Verification items for this drawing (mm, ordinates from the low corner). A direction names the side the tool comes from. Round coordinates to 2 decimals unless told otherwise and drop trailing zeros. Write each loop counter-clockwise with the first axis right and the second up, starting at its lowest first coordinate (ties: lowest second). Pieces come first, ordered by that corner, then holes. Notation, with made-up numbers: (-38.75, 71) -> (12.25, 71) arc R13 cw to (12.25, 94) -> close; hole circle Ø7 at (45.5, -5). An arc over 180 degrees is marked (long way). Put each result on its own line as item: value. Start each with the question number.
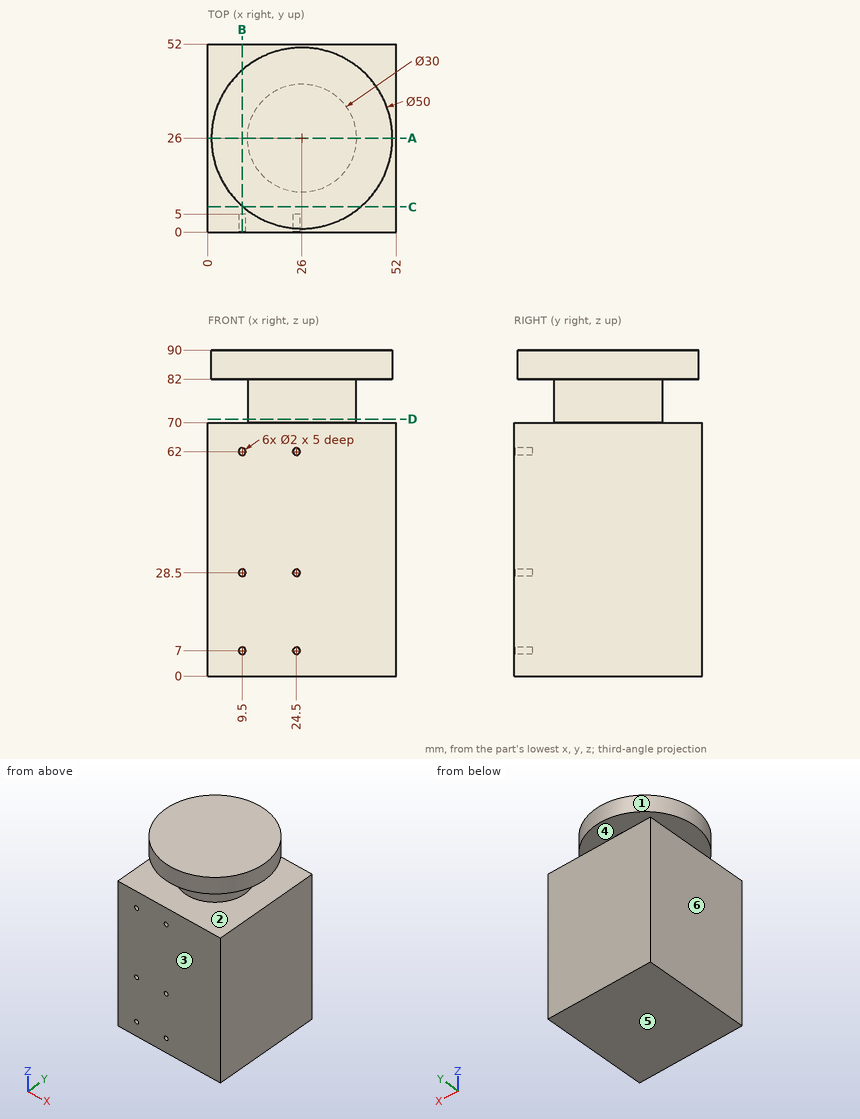
1. Access from +Z, -Z, +X, -X, +Y, -Y to the whole of each face (thin tool, end or side, straight path). Record for the marked faces 1, 2 and 3.
2. Gauge pin test, flat end, axial feed: P1, Ø1.6, axis at x = 9.5, z = 28.5, coming from the -Y side. Record the tip position at first contact, or that the pin passes through.
3. Section check C-C, the plane y = 7. Enter the section's corners in (x, z), then the cut area to 3 significant figures.
4. Draft check along Z on the marked faces 4, 5 and 6. Enter one of: released by +Z, released by -Z, zero draft, split by the parting line, or undercut.
5. Section check B-B, the plane x = 9.5. Enter the section's corners in (y, z).
6. Material ranges on L1, parallel to Z at x = 24.5, y = 2.75; L2, parallel to Z at x = 33, y = 7; L3, parallel to Z at x = 9.5, y = 2.8, recorded low to high. Write a range as [from, to].
7. Section check A-A, the plane y = 26. Enter the section's corners in (x, z), then the cut area to 3 significant figures.
8. Section check D-D, the plane z = 71. Enter the section's corners in (x, y), then the cut area to 3 significant figures.
Reply:
1. face 1: +Z
1. face 2: none
1. face 3: +Z, -Z, +X, -X, -Y
2. P1: stops at y = 5
3. outline: (0, 0) -> (52, 0) -> (52, 70) -> (0, 70) -> close; (9.75, 82) -> (42.25, 82) -> (42.25, 90) -> (9.75, 90) -> close
3. area: 3,900 mm2
4. face 4: undercut
4. face 5: released by -Z
4. face 6: zero draft
5. outline: (0, 0) -> (52, 0) -> (52, 70) -> (0, 70) -> (0, 63) -> (5, 63) -> (5, 61) -> (0, 61) -> (0, 29.5) -> (5, 29.5) -> (5, 27.5) -> (0, 27.5) -> (0, 8) -> (5, 8) -> (5, 6) -> (0, 6) -> close; (7.22, 82) -> (44.78, 82) -> (44.78, 90) -> (7.22, 90) -> close
6. L1: z = [0, 6], [8, 27.5], [29.5, 61], [63, 70], [82, 90]
6. L2: z = [0, 70], [82, 90]
6. L3: z = [0, 6], [8, 27.5], [29.5, 61], [63, 70]
7. outline: (0, 0) -> (52, 0) -> (52, 70) -> (41, 70) -> (41, 82) -> (51, 82) -> (51, 90) -> (1, 90) -> (1, 82) -> (11, 82) -> (11, 70) -> (0, 70) -> close
7. area: 4,400 mm2
8. outline: circle Ø30 at (26, 26)
8. area: 707 mm2
